Part model, mm, in its own coordinate system. Round coordinates to 2 decimals unless told otherwise and drop trailing zeros. Loops run counter-clockwise (first coordinate to the right, second up) from the corner with the lowest first, then second, coordinate; pieces in that order, holes last.
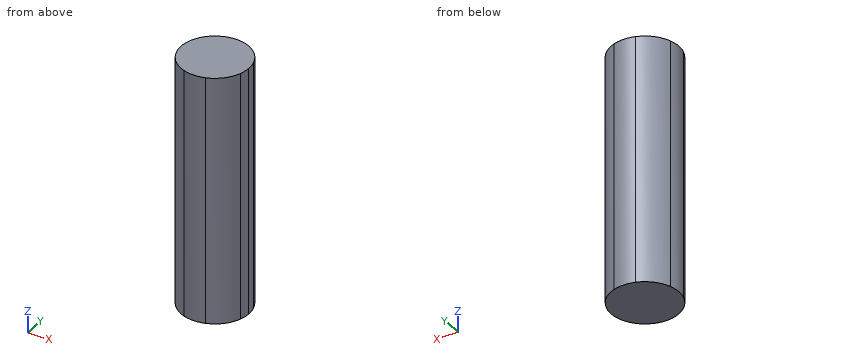
from build123d import *

# Parameters (mm, degrees)
F1_DEPTH = 46.0375


with BuildPart() as f1:
    # F0 (on Top) → F1 (new body)
    with BuildSketch(Plane.XY):
        with BuildLine():
            ThreePointArc((6, -2), (6.2428892318, -1.0130814572), (6.3245553203, 0))
            ThreePointArc((6.3245553203, 0), (6.2428892318, 1.0130814572), (6, 2))
            Line((6, 2), (6, -2))
        make_face()
        with BuildLine():
            Line((2, 2), (6, 2))
            ThreePointArc((6, 2), (4.472135955, 4.472135955), (2, 6))
            Line((2, 6), (2, 2))
        make_face()
        Polygon((6, -2), (6, 2), (2, 2), (2, 6), (-2, 6), (-2, 2), (-6, 2), (-6, -2), (-2, -2), (-2, -6), (2, -6), (2, -2), align=None)
        with BuildLine():
            ThreePointArc((2, -6), (4.472135955, -4.472135955), (6, -2))
            Line((6, -2), (2, -2))
            Line((2, -2), (2, -6))
        make_face()
        with BuildLine():
            Line((-2, 6), (2, 6))
            ThreePointArc((2, 6), (0, 6.3245553203), (-2, 6))
        make_face()
        with BuildLine():
            ThreePointArc((-2, -6), (0, -6.3245553203), (2, -6))
            Line((2, -6), (-2, -6))
        make_face()
        with BuildLine():
            Line((-2, 2), (-2, 6))
            ThreePointArc((-2, 6), (-4.472135955, 4.472135955), (-6, 2))
            Line((-6, 2), (-2, 2))
        make_face()
        with BuildLine():
            ThreePointArc((-6, -2), (-4.472135955, -4.472135955), (-2, -6))
            Line((-2, -6), (-2, -2))
            Line((-2, -2), (-6, -2))
        make_face()
        with BuildLine():
            Line((-6, -2), (-6, 2))
            ThreePointArc((-6, 2), (-6.3245553203, 0), (-6, -2))
        make_face()
    extrude(amount=F1_DEPTH)


solid = f1.part
1) Slice it at A-A, the plane z = 4. Give the cut face in (x, y), then the cut area to 3 significant figures.
Values:
outline: circle Ø12.65 at (0, 0)
area: 126 mm2
2) Wall check: line 1 along X through (y, z) = (2, 30.5); line 2 along X through (y, z) = (-5.5, 4). Give the ranges that are in metal, low to high.
Values:
line 1: x = -6 to 6
line 2: x = -3.12 to 3.12
3) Slice it at C-C, the plane y = -3.25. Give the cut face in (x, z), then the cut area to 3 significant figures.
Values:
outline: (-5.43, 0) - (5.43, 0) - (5.43, 46.04) - (-5.43, 46.04) - close
area: 500 mm2
4) Slice it at B-B, the plane x = -3.5. Give the cut face in (y, z).
Values:
outline: (-5.27, 0) - (5.27, 0) - (5.27, 46.04) - (-5.27, 46.04) - close
5) Drop flat-ended pins along their axis: pin 1 Ø2 at (x, z) = (1.5, 40) entering from +Y; pin 2 Ø1.5 at (x, z) = (1, 41) entering from -Y; pin 3 Ø2 at (y, z) = (-1.5, 40) entering from +X. Give the stop position or say it passes through.
Values:
pin 1: stops at y = 6.3
pin 2: stops at y = -6.32
pin 3: stops at x = 6.3
